The model under review builds one solid part; all positions refer to its coordinate system, in mm. A direction names the side the tool comes from. Round coordinates to 2 decimals unless told otherwise and drop trailing zeros. Write each loop counter-clockwise with the first axis right and the second up, starting at its lowest first coordinate (ties: lowest second). Pieces come first, ordered by that corner, then holes. Notation, with made-up numbers: (-35.75, 12.25) - (-21.75, 12.25) arc R28 ccw to (-21.75, 35.25) - close; hole circle Ø8 at (-16.75, -5). An arc over 180 degrees is marked (long way). Return JSON: item names as keys, results as strings.
Autodesk Inventor part; units mm, degrees
ref_plane "YZ Plane" through (0, 0, 0) normal (1, 0, 0) x (0, 1, 0)
ref_plane "XZ Plane" through (0, 0, 0) normal (0, 1, 0) x (-1, 0, 0)
ref_plane "XY Plane" through (0, 0, 0) normal (0, 0, 1) x (1, 0, 0)
sketch "Sketch1" plane through (0, 0, 0) normal (0, 1, 0) x (-1, 0, 0)
  line L0 (40.7087, 37.7886) -> (-28.4413, 37.7886)
  line L1 (-28.4413, 37.7886) -> (-28.4413, -50.4114)
  line L2 (-28.4413, -50.4114) -> (40.7087, -50.4114)
  line L3 (40.7087, -50.4114) -> (40.7087, 37.7886)
  point P0 (0, 0)
  dimension "d0" = 88.2
  dimension "d1" = 69.15
extrude "Extrusion1" add sketch "Sketch1" along normal blind 3
sketch "Sketch2" plane through (0, 3, 0) normal (0, 1, 0) x (1, 0, 0)
  line L0 (-40.7087, -37.7886) -> (28.4413, -37.7886)
  line L1 (28.4413, -37.7886) -> (28.4413, 50.4114)
  line L2 (-40.7087, -37.7886) -> (28.4413, -37.7886)
  line L3 (28.4413, -37.7886) -> (28.4413, -32.7886)
  line L4 (28.4413, -32.7886) -> (-40.7087, -32.7886)
  line L5 (-40.7087, -32.7886) -> (-40.7087, -37.7886)
  line L6 (-40.7087, 50.4114) -> (-40.7087, -37.7886)
  line L7 (-40.7087, -37.7886) -> (-35.7087, -37.7886)
  line L8 (-35.7087, -37.7886) -> (-35.7087, 50.4114)
  line L9 (-35.7087, 50.4114) -> (-40.7087, 50.4114)
  line L10 (-40.7087, 50.4114) -> (-40.7087, -37.7886)
  line L11 (28.4413, 50.4114) -> (-40.7087, 50.4114)
  line L12 (-40.7087, 45.4114) -> (28.4413, 45.4114)
  line L13 (28.4413, 45.4114) -> (28.4413, 50.4114)
  line L14 (28.4413, 50.4114) -> (-40.7087, 50.4114)
  line L15 (-40.7087, 50.4114) -> (-40.7087, 45.4114)
  line L16 (28.4413, 50.4114) -> (23.4413, 50.4114)
  line L17 (23.4413, 50.4114) -> (23.4413, -37.7886)
  line L18 (23.4413, -37.7886) -> (28.4413, -37.7886)
  line L19 (28.4413, -37.7886) -> (28.4413, 50.4114)
  point P0 (0, 0)
  dimension "d4" = 5
  dimension "d5" = 5
  dimension "d6" = 5
  dimension "d7" = 5
extrude "Extrusion2" add sketch "Sketch2" along normal blind 13 contours L5 L4 L8 L0 | L8 L4 L17 L0 | L6 L12 L8 L4 | L17 L4 L1 L0 | L6 L9 L8 L12 | L17 L12 L1 L4 | L8 L11 L17 L12 | L17 L11 L1 L12
fillet "Fillet1" radius 10 4 edges at (28.4413, 8, 37.7886) (28.4413, 8, -50.4114) (-40.7087, 8, 37.7886) (-40.7087, 8, -50.4114)
sketch "Sketch3" plane through (0, 3, 0) normal (0, 1, 0) x (1, 0, 0)
  line L0 (-35.7087, -32.7886) -> (23.4413, -32.7886)
  line L1 (-35.7087, -32.7886) -> (-29.7087, -32.7886)
  line L2 (-29.7087, -32.7886) -> (-29.7087, -26.7886)
  line L3 (-29.7087, -26.7886) -> (-35.7087, -26.7886)
  line L4 (-35.7087, -26.7886) -> (-35.7087, -32.7886)
  line L5 (-35.7087, 45.4114) -> (-35.7087, -32.7886)
  line L6 (-35.7087, 45.4114) -> (-29.7087, 45.4114)
  line L7 (-29.7087, 45.4114) -> (-29.7087, 39.4114)
  line L8 (-29.7087, 39.4114) -> (-35.7087, 39.4114)
  line L9 (-35.7087, 39.4114) -> (-35.7087, 45.4114)
  line L10 (23.4413, -32.7886) -> (23.4413, 45.4114)
  line L11 (23.4413, 45.4114) -> (17.4413, 45.4114)
  line L12 (17.4413, 45.4114) -> (17.4413, 39.4114)
  line L13 (17.4413, 39.4114) -> (23.4413, 39.4114)
  line L14 (23.4413, 39.4114) -> (23.4413, 45.4114)
  line L15 (23.4413, -32.7886) -> (17.4413, -32.7886)
  line L16 (17.4413, -32.7886) -> (17.4413, -26.7886)
  line L17 (17.4413, -26.7886) -> (23.4413, -26.7886)
  line L18 (23.4413, -26.7886) -> (23.4413, -32.7886)
  point P0 (0, 0)
  dimension "d11" = 6
  dimension "d12" = 6
  dimension "d13" = 6
  dimension "d14" = 6
  dimension "d15" = 6
  dimension "d16" = 6
  dimension "d17" = 6
  dimension "d18" = 6
extrude "Extrusion3" add sketch "Sketch3" along normal up to surface (13 mm away)
fillet "Fillet2" radius 3 4 edges at (-29.7087, 9.5, -39.4114) (-29.7087, 9.5, 26.7886) (17.4413, 9.5, -39.4114) (17.4413, 9.5, 26.7886)
sketch "Sketch4" plane through (0, 16, 0) normal (0, 1, 0) x (1, 0, 0)
  line L0 (28.4413, -27.7886) -> (28.4413, 40.4114)
  line L1 (-30.7087, -37.7886) -> (18.4413, -37.7886)
  line L2 (-40.7087, 40.4114) -> (-40.7087, -27.7886)
  line L3 (18.4413, 50.4114) -> (-30.7087, 50.4114)
  point P0 (0, 0)
  point P1 (21.4413, -30.7886)
  point P2 (-33.7087, -30.7886)
  point P3 (-33.7087, 43.4114)
  point P4 (21.4413, 43.4114)
  dimension "d22" = 7
  dimension "d23" = 7
  dimension "d24" = 7
  dimension "d25" = 7
  dimension "d26" = 7
  dimension "d27" = 7
  dimension "d28" = 7
  dimension "d29" = 7
hole "Hole1" at (21.4413, 16, 30.7886) at (-33.7087, 16, 30.7886) at (-33.7087, 16, -43.4114) at (21.4413, 16, -43.4114) direction (0, -1, 0) diameter 3 depth 6
sketch "Sketch5" plane through (-35.7087, 3, 26.7886) normal (1, 0, 0) x (0, 0, -1)
  line L0 (66.2, 0) -> (0, 0)
  line L1 (28, 0) -> (38.2, 0)
  line L2 (38.2, 0) -> (38.2, 4)
  line L3 (38.2, 4) -> (28, 4)
  line L4 (28, 4) -> (28, 0)
  line L5 (0, 13) -> (0, 0)
  point P0 (26.7886, -3)
  point P1 (66.2, 13)
  dimension "d37" = 4
  dimension "d38" = 10.2
  dimension "d39" = 28
  dimension "d40" = 28
  dimension "d41" = 66.2
extrude "Extrusion4" cut sketch "Sketch5" against normal blind 13
sketch "Sketch6" plane through (-40.7087, 0, -40.4114) normal (-1, 0, 0) x (0, 0, 1)
  line L0 (26, 10) -> (42.2, 10)
  line L1 (42.2, 10) -> (42.2, 0)
  line L2 (42.2, 0) -> (26, 0)
  line L3 (26, 0) -> (26, 10)
  line L4 (39.2, 7) -> (39.2, 3)
  line L5 (29, 3) -> (29, 7)
  line L6 (39.2, 3) -> (29, 3)
  line L7 (29, 7) -> (39.2, 7)
  point P0 (40.4114, 0)
  dimension "d44" = 3
  dimension "d45" = 3
  dimension "d46" = 3
  dimension "d47" = 3
extrude "Extrusion5" cut sketch "Sketch6" against normal blind 3
sketch "Sketch7" plane through (-35.7087, 3, -39.4114) normal (1, 0, 0) x (0, 0, -1)
  line L0 (-38.2, 0) -> (-66.2, 0)
  line L1 (-43.1, 0) -> (-23.1, 0)
  line L2 (-23.1, 0) -> (-23.1, 300)
  line L3 (-23.1, 300) -> (-43.1, 300)
  line L4 (-43.1, 300) -> (-43.1, 0)
  line L5 (-28, 4) -> (-28, 0)
  line L6 (-38.2, 0) -> (-38.2, 4)
  point P0 (-39.4114, -3)
  dimension "d50" = 20
  dimension "d51" = 4.9
  dimension "d52" = 4.9
  dimension "d53" = 10.2
  dimension "d102" = 300
extrude "Extrusion6" cut sketch "Sketch7" against normal blind 2
sketch "Sketch8" plane through (0, 3, 0) normal (0, 1, 0) x (1, 0, 0)
  line L0 (-37.7087, 16.3114) -> (-37.7087, 14.4114)
  line L1 (-37.7087, 16.3114) -> (-2.7087, 16.3114)
  line L2 (-2.7087, 16.3114) -> (-2.7087, -3.6886)
  line L3 (-2.7087, -3.6886) -> (-37.7087, -3.6886)
  line L4 (-37.7087, -3.6886) -> (-37.7087, 16.3114)
  line L5 (-35.7087, -3.6886) -> (-37.7087, -3.6886)
  point P0 (0, 0)
  dimension "d56" = 20
  dimension "d57" = 20
  dimension "d58" = 35
extrude "Extrusion7" cut sketch "Sketch8" against normal blind 1
sketch "Sketch14" plane through (0, 3, 0) normal (0, 1, 0) x (1, 0, 0)
  line L0 (-27.7087, -26.7886) -> (-21.5087, -26.7886)
  line L1 (-21.5087, -26.7886) -> (-21.5087, -20.5886)
  line L2 (-21.5087, -20.5886) -> (-27.7087, -20.5886)
  line L3 (-27.7087, -20.5886) -> (-27.7087, -26.7886)
  line L4 (17.4413, -32.7886) -> (-29.7087, -32.7886)
  line L5 (-35.7087, -26.7886) -> (-35.7087, -3.6886)
  point P0 (0, 0)
  dimension "d103" = 6.2
  dimension "d104" = 6
  dimension "d105" = 8
  dimension "d106" = 6.2
extrude "Extrusion11" cut sketch "Sketch14" against normal blind 1
sketch "Sketch15" plane through (0, 2, 0) normal (0, 1, 0) x (1, 0, 0)
  circle A0 centre (-24.6087, -23.6886) radius 1.875
  line L0 (-21.5087, -20.5886) -> (-21.5087, -26.7886)
  line L1 (-27.7087, -26.7886) -> (-27.7087, -20.5886)
  line L2 (-27.7087, -20.5886) -> (-21.5087, -20.5886)
  line L3 (-21.5087, -26.7886) -> (-27.7087, -26.7886)
  point P0 (0, 0)
  dimension "d109" = 3.1
  dimension "d110" = 3.1
  dimension "d111" = 3.1
  dimension "d112" = 3.1
  dimension "d113" = 3.75
extrude "Extrusion12" cut sketch "Sketch15" against normal through all contours A0
equation "\"d5\" = d4"
equation "\"d6\" = d4"
equation "\"d7\" = d4"
equation "\"d11\" = d12"
equation "\"d13\" = d12"
equation "\"d14\" = d13"
equation "\"d15\" = d13"
equation "\"d16\" = d15"
equation "\"d17\" = d15"
equation "\"d18\" = d17"
equation "\"d45\" = d44"
equation "\"d47\" = d44"
equation "\"d51\" = -0.5 * d53 + 0.5 * d50"
equation "\"d56\" = d57"
equation "\"d103\" = d106"
equation "\"d109\" = d112"
properties part number "macropad-frame"
(1) Add section C-C (z = 18.5). Write out the cut boundary in (x, y).
Filled in:
{"outline": "(-40.71, 0) - (28.44, 0) - (28.44, 16) - (23.44, 16) - (23.44, 3) - (-35.71, 3) - (-35.71, 16) - (-40.71, 16) - close"}
(2) For faces 1 (the flat face through (-39, 5, -14.411)), 2 (the flat face through (-25.3, 2.7, -16.311)), 3 (the cylindrical face through (25.43, 8.11, 34.94)), list the 3-axis set-ups (+Z, -Z, +X, -X, +Y, -Y) from which the entire face can be reached by the end or side of a thin tool; tool diameter is ignored.
Filled in:
{"face 1": "-X, -Y", "face 2": "+Y", "face 3": "+Z, +X, +Y, -Y"}
(3) Mouldability with a two-part tool opening along Z and no side actions: class faces 4 (the cylindrical face through (-26.482, 1.014, 23.606)), 5 (the flat face through (-6, 8, 37.789)) as released by +Z, released by -Z, zero draft, split by the parting line, or undercut.
Filled in:
{"face 4": "undercut", "face 5": "released by +Z"}
(4) Add section B-B (y = 13). Give the number of separate pieces and of enclosed holes in the cut face, plus the area to 3 significant figures.
Filled in:
{"separate pieces": "1", "enclosed holes": "5", "area": "1,460 mm2"}
(5) Wall thickness on line 1 (X direction, y = 11, z = -32); line 2 (Z direction, x = -32.5, y = 12); line 3 (X direction, y = 13.25, z = 31): over which ranges is each line inside the solid? List them lowest first.
Filled in:
{"line 1": "x = -40.71 to -35.71, 23.44 to 28.44", "line 2": "z = -50.25 to -44.3, -42.52 to -39.42, 26.8 to 29.9, 31.68 to 37.63", "line 3": "x = -40.18 to -35.19, -32.22 to -29.71, 17.44 to 19.96, 22.93 to 27.91"}
(6) Add section A-A (x = -20.5). Write out the cut boundary in (y, z), plus the area to 3 significant figures.
Filled in:
{"outline": "(0, -50.41) - (16, -50.41) - (16, -45.41) - (3, -45.41) - (3, -16.31) - (2, -16.31) - (2, 3.69) - (3, 3.69) - (3, 32.79) - (16, 32.79) - (16, 37.79) - (0, 37.79) - close", "area": "375 mm2"}
(7) Clearance check with flat-ended pins moving along their axes: pin 1 Ø8 at (x, z) = (-27.5, -12) entering from +Y; pin 2 Ø1.5 at (x, z) = (-33.5, -42.5) entering from +Y; pin 3 Ø16 at (x, z) = (-13, -10) entering from +Y; pin 4 Ø2 at (y, z) = (1, -6) entering from -X. State where each tip first meets the part, or that it passes through.
Filled in:
{"pin 1": "stops at y = 2", "pin 2": "stops at y = 16", "pin 3": "stops at y = 3", "pin 4": "stops at x = -37.71"}
